Check sheet for the modelled part. Datum: model origin and axes. Units: mm. Face numbers are marked on the shaded views. A direction names the side the tool comes from. Round coordinates to 2 decimals unless told otherwise and drop trailing zeros. Write each loop counter-clockwise with the first axis right and the second up, starting at its lowest first coordinate (ties: lowest second). Pieces come first, ordered by that corner, then holes. Notation, with made-up numbers: M 31,23 L 77,23 A28 ccw 77,50 Z; hole C -32.5,34.5 d11. An arc over 180 degrees is marked long. Answer in a Markdown table with one row per item.
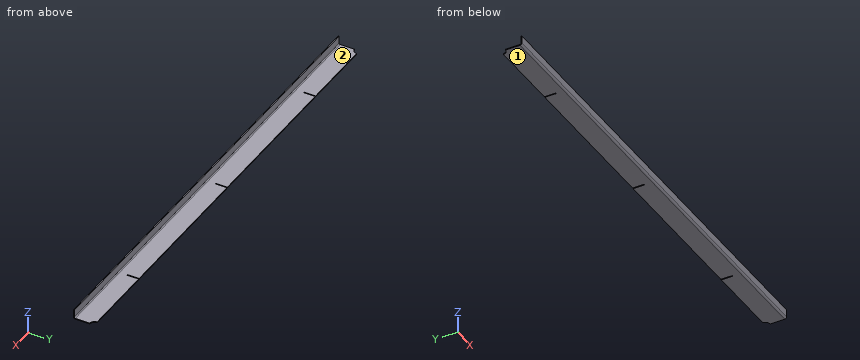
Autodesk Inventor part; units mm, degrees
ref_plane "YZ Plane" through (0, 0, 0) normal (1, 0, 0) x (0, 1, 0)
ref_plane "XZ Plane" through (0, 0, 0) normal (0, 1, 0) x (-1, 0, 0)
ref_plane "XY Plane" through (0, 0, 0) normal (0, 0, 1) x (1, 0, 0)
sketch "Sketch1" plane through (0, 0, 0) normal (0, 0, 1) x (1, 0, 0)
  line L0 (-750, 67.5235) -> (750, 67.5235)
  line L1 (750, 67.5235) -> (750, 0)
  line L2 (750, 0) -> (-750, 0)
  line L3 (-750, 0) -> (-750, 67.5235)
  point P0 (0, 0)
  point P1 (0, 0)
  dimension "d0" = 1500
  dimension "d1" = 67.5235
extrude "Plate1" add sketch "Sketch1" along normal blind 3
sketch "Sketch2" plane through (750, 3, 0) normal (0, -1, 0) x (1, 0, 0)
  line L0 (-1500, 0) -> (0, 0)
  line L1 (0, 0) -> (0, 30)
  line L2 (0, 30) -> (-1500, 30)
  line L3 (-1500, 30) -> (-1500, 0)
edge flange "Flange1" height 30 angle 90 thickness 3 bend radius 3 thickness toward (0, -1, 0) relief tear relief width 3 relief depth 1.5 edges at (0, 0, 3) wall of the first edge with corners at (-750, 3, 0) (750, 3, 0) (750, 3, 30) (-750, 3, 30)
bend "Bend1"
corner "Corner1"
sketch "Sketch5" plane through (0, 0, 0) normal (0, 0, -1) x (-1, 0, 0)
  line L0 (750, 67.5235) -> (-750, 67.5235)
  line L1 (500, 67.5235) -> (500, 31)
  line L2 (500, 31) -> (503, 31)
  line L3 (503, 31) -> (503, 67.5235)
  line L4 (750, 0) -> (-750, 0)
  point P0 (0, 0)
  dimension "d18" = 3
  dimension "d19" = 247
  dimension "d20" = 31
extrude "Extrusion1" cut sketch "Sketch5" against normal through all
pattern_linear "Rectangular Pattern1" count 3 spacing 500 along (1, 0, 0) of "Extrusion1"
sketch "Sketch6" plane through (0, 0, 0) normal (0, 0, -1) x (-1, 0, 0)
  line L0 (-750, 67.5235) -> (-750, 6)
  circle A0 centre (-750, 67.5235) radius 15
  line L1 (-750, 67.5235) -> (750, 67.5235)
  point P0 (0, 0)
  point P1 (-500, 67.5235)
  point P2 (-735, 67.5235)
  point P3 (-750, 52.5235)
  dimension "d24" = 30
extrude "Extrusion2" cut sketch "Sketch6" against normal through all contours L1 A0 L0 picked at (-740.1254, 66.4109)
mirror "Mirror1" about plane through (0, 0, 0) normal (1, 0, 0) of "Extrusion2"
equation "\"d1\" = Стрингер_3"
equation "\"d18\" = Thickness"
equation "\"d2\" = Thickness"
equation "\"d3\" = BendReliefWidth"
equation "\"d4\" = BendReliefDepth"
equation "\"d5\" = MinimumRemnant"
equation "\"d6\" = TransitionRadius"
equation "\"d9\" = BendRadius"
equation "\"d10\" = CornerReliefSize"
equation "\"d11\" = GapSize"
equation "\"d12\" = JacobiRadiusSize"
equation "\"BendRadius\" = Thickness"
equation "\"BendReliefWidth\" = Thickness"
equation "\"BendReliefDepth\" = 0.5 * Thickness"
equation "\"CornerReliefSize\" = 4 * Thickness"
equation "\"MinimumRemnant\" = 2 * Thickness"
equation "\"TransitionRadius\" = BendRadius"
equation "\"JacobiRadiusSize\" = BendRadius"
equation "\"GapSize\" = Thickness"
properties part number "МОО 053 стрингер борт 31"
1. Go/stop test with flat-tipped pins: pin 1 (1.5 mm diameter, centred on y = 56, z = 2, fed in from +X); pin 2 (18.5 mm diameter, centred on x = -261.5, y = 30.5, fed in from +Z); pin 3 (0.9 mm diameter, centred on x = 498, z = 2, fed in from +Y). Record where each tip stops, or that it passes through.
Found:
| item | result |
|---|---|
| pin 1 | stops at x = 741.38 |
| pin 2 | stops at z = 3 |
| pin 3 | stops at y = 31 |
2. Access from +Z, -Z, +X, -X, +Y, -Y to the whole of each face (thin tool, end or side, straight path). Record for the marked faces 1 and 2.
Found:
| item | result |
|---|---|
| face 1 | -Z, +X, -X, +Y, -Y |
| face 2 | +Z, +X, -X, +Y |
3. Section check A-A, the plane x = 234. Record the cut outline in (y, z), and give its area (3 significant figures).
Found:
| item | result |
|---|---|
| outline | M 0,6 A6 ccw 6,0 L 67.52,0 L 67.52,3 L 6,3 A3 cw 3,6 L 3,30 L 0,30 Z |
| area | 278 mm2 |
4. Scan lines: L1, parallel to Z at x = 318, y = 16; L2, parallel to Y at x = -131, z = 3.75. Record each from-to range of solid material in increasing order.
Found:
| item | result |
|---|---|
| L1 | z = 0 to 3 |
| L2 | y = 0.44 to 4.02 |
5. Section check B-B, the plane z = 21. Record the cut outline in (x, y), and give its area (3 significant figures).
Found:
| item | result |
|---|---|
| outline | M -750,0 L 750,0 L 750,3 L -750,3 Z |
| area | 4,500 mm2 |
